Design review of the part shown in the three views and the two pictorial views. Dimensions are in mm from the part's minimum x, y and z. Give positions to 0.01 mm unless a question says otherwise; leave off trailing zeros. Order: outer loops, then holes, each group sorted by start corner. A loop starts at its lowest first (then second) coordinate and runs counter-clockwise, first axis right, second up.
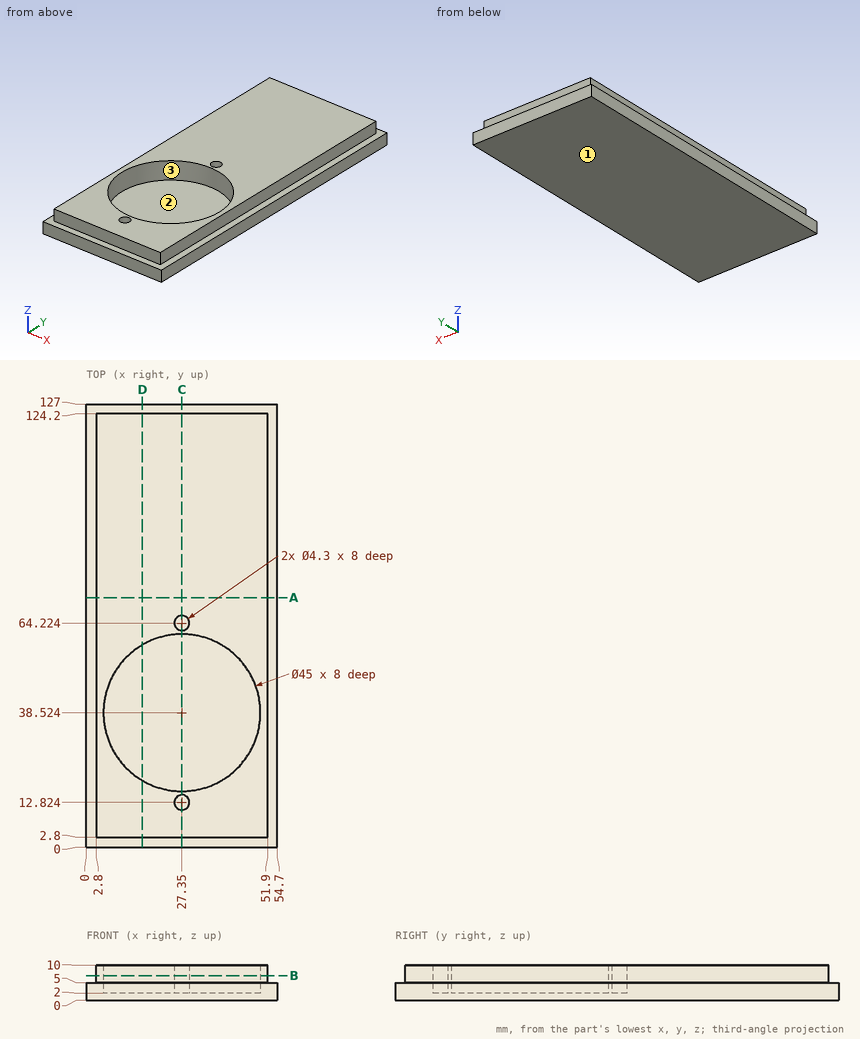
1) To check wall thickness, follow line 1 (Y direction, x = 27.35, z = 6.25); line 2 (Y direction, x = 27.35, z = 3.75); line 3 (X direction, y = 23.5, z = 5.75). State the ranges of each line that lie inside material, in increasing order.
Answer sheet:
line 1: y = 2.8 to 10.67, 14.97 to 16.02, 61.02 to 62.07, 66.37 to 124.2
line 2: y = 0 to 10.67, 14.97 to 16.02, 61.02 to 62.07, 66.37 to 127
line 3: x = 2.8 to 10.6, 44.1 to 51.9
2) Clearance check with flat-ended pins moving along their axes: pin 1 (2.5 mm diameter, centred on x = 31, z = 7, fed in from +Y); pin 2 (2.5 mm diameter, centred on y = 59.5, z = 8.5, fed in from +X); pin 3 (2.5 mm diameter, centred on y = 58, z = 7, fed in from -X). State where each tip first meets the part, or that it passes through.
Answer sheet:
pin 1: stops at y = 124.2
pin 2: stops at x = 51.9
pin 3: stops at x = 2.8
3) We need section C-C on x = 27.35. Give the boundary of the cut face in (y, z), then the cut area to 3 significant figures.
Answer sheet:
outline: (0, 0) - (127, 0) - (127, 5) - (124.2, 5) - (124.2, 10) - (66.37, 10) - (66.37, 2) - (62.07, 2) - (62.07, 10) - (61.02, 10) - (61.02, 2) - (16.02, 2) - (16.02, 10) - (14.97, 10) - (14.97, 2) - (10.67, 2) - (10.67, 10) - (2.8, 10) - (2.8, 5) - (0, 5) - close
area: 813 mm2
4) We need section D-D on x = 16. Give the boundary of the cut face in (y, z), then the cut area to 3 significant figures.
Answer sheet:
outline: (0, 0) - (127, 0) - (127, 5) - (124.2, 5) - (124.2, 10) - (57.95, 10) - (57.95, 2) - (19.1, 2) - (19.1, 10) - (2.8, 10) - (2.8, 5) - (0, 5) - close
area: 931 mm2
5) Draft analysis for pull direction Y (two halves, no side actions). For the marked faces 1, 2 and 3, state which applies: +Y half, -Y half, draft (parallel to the pull), parting line (faces both ways), or undercut.
Answer sheet:
face 1: draft
face 2: undercut
face 3: undercut
6) We need section B-B on z = 7. Give the boundary of the cut face in (x, y), then the cut area to 3 significant figures.
Answer sheet:
outline: (2.8, 2.8) - (51.9, 2.8) - (51.9, 124.2) - (2.8, 124.2) - close; hole circle Ø45 at (27.35, 38.52); hole circle Ø4.3 at (27.35, 12.82); hole circle Ø4.3 at (27.35, 64.22)
area: 4,340 mm2
7) We need section A-A on y = 71.5. Give the boundary of the cut face in (x, z), then the cut area to 3 significant figures.
Answer sheet:
outline: (0, 0) - (54.7, 0) - (54.7, 5) - (51.9, 5) - (51.9, 10) - (2.8, 10) - (2.8, 5) - (0, 5) - close
area: 519 mm2
